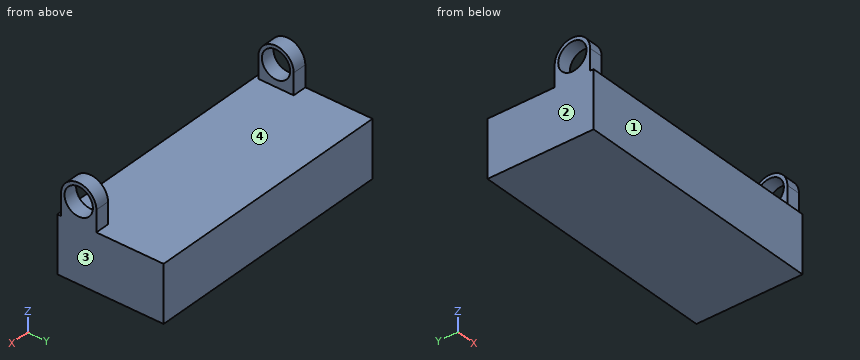
from build123d import *

# Parameters (mm, degrees)
ESQUISSE1_W                = 36
ESQUISSE1_H                = 15
BOSS_EXTRU_3_DEPTH         = 8
ESQUISSE2_R                = 2
BOSS_EXTRU_4_DEPTH         = 2
R_P_TITION_LIN_AIRE1_COUNT = 2
R_P_TITION_LIN_AIRE1_PITCH = 34


with BuildPart() as part:
    # Esquisse1 → Boss.-Extru.3 (new body)
    with BuildSketch(Plane.XY):
        with Locations((18, 7.5)):
            Rectangle(ESQUISSE1_W, ESQUISSE1_H)
    extrude(amount=BOSS_EXTRU_3_DEPTH)

    # Esquisse2 → Boss.-Extru.4 (add)
    with BuildSketch(Plane.ZY):
        with BuildLine():
            Line((11, 5.5), (8, 5.5))
            Line((8, 5.5), (8, 0.5))
            Line((8, 0.5), (11, 0.5))
            ThreePointArc((11, 0.5), (13.5, 3), (11, 5.5))
        make_face()
        with Locations((11, 3)):
            Circle(ESQUISSE2_R, mode=Mode.SUBTRACT)
    boss_extru_4 = extrude(amount=-BOSS_EXTRU_4_DEPTH)

    # Répétition linéaire1: Boss.-Extru.4 ×2
    with Locations(*[(i * R_P_TITION_LIN_AIRE1_PITCH, 0, 0) for i in range(1, R_P_TITION_LIN_AIRE1_COUNT)]):
        add(boss_extru_4)


solid = part.part
Model file for the job. Use its own axes, mm. Face numbers are marked on the shaded views. Give positions to 0.01 mm unless a question says otherwise; leave off trailing zeros. Loops run counter-clockwise (first coordinate to the right, second up) from the corner with the lowest first, then second, coordinate; pieces in that order, holes last. Notation, with made-up numbers: (51, -23.75) - (98, -23.75) arc R15 cw to (98, -9.75) - close; hole circle Ø9 at (75.5, 85). An arc over 180 degrees is marked (long way). Use one line per item in the form item = value.
(1) Cut at B-B (x = 27.5). Give the cut face in (y, z), then the cut area to 3 significant figures.
Determined:
outline = (0, 0) - (15, 0) - (15, 8) - (0, 8) - close
area = 120 mm^2
(2) Cut at A-A (y = 3). Give the cut face in (x, z).
Determined:
outline = (0, 0) - (36, 0) - (36, 9) - (34, 9) - (34, 8) - (2, 8) - (2, 9) - (0, 9) - close; (0, 13) - (2, 13) - (2, 13.5) - (0, 13.5) - close; (34, 13) - (36, 13) - (36, 13.5) - (34, 13.5) - close
(3) Cut at C-C (y = 7.5). Give the cut face in (x, z), then the cut area to 3 significant figures.
Determined:
outline = (0, 0) - (36, 0) - (36, 8) - (0, 8) - close
area = 288 mm^2
(4) Drill centre lines: L1, parallel to Y at x = 34.85, z = 11; L2, parallel to Z at x = 2.5, y = 10.75. Where is each one in solid material? Low to high.
Determined:
L1 = 0.5 to 1, 5 to 5.5
L2 = 0 to 8
(5) Pull direction X, two halves, no side cores. Call the marked faces 1, 2, 3 and 4: pulls with the +X half, pulls with the -X half, needs draft (parallel to the pull), parting line crosses it, or undercut.
Determined:
face_1 = needs draft
face_2 = pulls with the -X half
face_3 = pulls with the +X half
face_4 = undercut
(6) Drop flat-ended pins along their axis: P1, Ø1, axis at x = 0.5, z = 9.5, coming from the +Y side; P2, Ø4, axis at x = 22.5, y = 13, coming from the +Z side; P3, Ø1.6, axis at x = 35, z = 10, coming from the -Y side. Give the stop position or say it passes through.
Determined:
P1 = 5.5
P2 = 8
P3 = 0.5
